from build123d import *

# Parameters (mm, degrees)
ESQUISSE1_W        = 72.2
ESQUISSE1_H        = 67.82
ESQUISSE1_R        = 1.5
BOSS_EXTRU_1_DEPTH = 1.5
ESQUISSE1_4_W      = 72.2
ESQUISSE1_4_H      = 67.82
ESQUISSE1_4_R      = 1.5
ESQUISSE1_4_W_2    = 60
ESQUISSE1_4_H_2    = 30
BOSS_EXTRU_2_DEPTH = 1.5


with BuildPart() as part:
    # Esquisse1 → Boss.-Extru.1 (new body)
    with BuildSketch(Plane(origin=(0, 0, 0), x_dir=(1, 0, 0), z_dir=(0, 1, 0))):
        Rectangle(ESQUISSE1_W, ESQUISSE1_H)
        with Locations(Location((-32.2, 30.41, 0), (0, 0, 270))):
            Circle(ESQUISSE1_R, mode=Mode.SUBTRACT)
        with Locations(Location((32.8, 30.41, 0), (0, 0, 270))):
            Circle(ESQUISSE1_R, mode=Mode.SUBTRACT)
        with Locations(Location((-32.2, -29.59, 0), (0, 0, 270))):
            Circle(ESQUISSE1_R, mode=Mode.SUBTRACT)
        with Locations(Location((32.8, -29.59, 0), (0, 0, 270))):
            Circle(ESQUISSE1_R, mode=Mode.SUBTRACT)
    extrude(amount=BOSS_EXTRU_1_DEPTH)

    # Esquisse1_4 → Boss.-Extru.2 (add)
    with BuildSketch(Plane(origin=(0, 0, 0), x_dir=(1, 0, 0), z_dir=(0, 1, 0))):
        Rectangle(ESQUISSE1_4_W, ESQUISSE1_4_H)
        with Locations(Location((-32.2, 30.41, 0), (0, 0, 270))):
            Circle(ESQUISSE1_4_R, mode=Mode.SUBTRACT)
        with Locations(Location((32.8, 30.41, 0), (0, 0, 270))):
            Circle(ESQUISSE1_4_R, mode=Mode.SUBTRACT)
        with Locations(Location((-32.2, -29.59, 0), (0, 0, 270))):
            Circle(ESQUISSE1_4_R, mode=Mode.SUBTRACT)
        with Locations(Location((32.8, -29.59, 0), (0, 0, 270))):
            Circle(ESQUISSE1_4_R, mode=Mode.SUBTRACT)
        with Locations((-0.3, 3.91)):
            Rectangle(ESQUISSE1_4_W_2, ESQUISSE1_4_H_2, mode=Mode.SUBTRACT)
    extrude(amount=BOSS_EXTRU_2_DEPTH)


solid = part.part
The listing builds one solid part. Answer for the finished solid, in the listing's coordinates (mm). Coordinates: 2 decimals unless noted, no trailing zeros. Loops run counter-clockwise (first coordinate to the right, second up) from the corner with the lowest first, then second, coordinate; pieces in that order, holes last.
1) Determine the mould class of faces 1 (the face through (-1, 0, 0)), 2 (the face through (36.1, 1, 0)), 3 (the face through (-36.1, 1, 0)), 4 (the face through (-30.935, 0.74, -29.604)) for opening direction X: pulls with the +X half, pulls with the -X half, needs draft (parallel to the pull), parting line crosses it, or undercut.
2) Find the intervals of material crossed by L1, parallel to X at y = 0.9, z = 29.59, in increasing order.
3) Find section B-B on x = -32.2. Write down the section's boundary in (y, z), then the cut area to 3 significant figures.
4) Find section A-A on z = -30.41. Write down the section's boundary in (x, y), then the cut area to 3 significant figures.
Values:
1. face 1: needs draft
1. face 2: pulls with the +X half
1. face 3: pulls with the -X half
1. face 4: undercut
2. L1: x = -36.1 to -33.7, -30.7 to 31.3, 34.3 to 36.1
3. outline: (0, -33.91) - (1.5, -33.91) - (1.5, -31.91) - (0, -31.91) - close; (0, -28.91) - (1.5, -28.91) - (1.5, 28.09) - (0, 28.09) - close; (0, 31.09) - (1.5, 31.09) - (1.5, 33.91) - (0, 33.91) - close
3. area: 92.7 mm2
4. outline: (-36.1, 0) - (-33.7, 0) - (-33.7, 1.5) - (-36.1, 1.5) - close; (-30.7, 0) - (31.3, 0) - (31.3, 1.5) - (-30.7, 1.5) - close; (34.3, 0) - (36.1, 0) - (36.1, 1.5) - (34.3, 1.5) - close
4. area: 99.3 mm2
